For this review, take the finished solid that the model builds, in its own axes (mm). Face numbers are marked on the shaded views. Round coordinates to 2 decimals unless told otherwise and drop trailing zeros. Order: outer loops, then holes, each group sorted by start corner. A loop starts at its lowest first (then second) coordinate and runs counter-clockwise, first axis right, second up. Notation, with made-up numbers: M -31.75,18.25 L -9.75,18.25 A16 cw -9.75,34.25 Z; hole C 37,36 d3. An arc over 180 degrees is marked long. Answer in a Markdown table with one row per item. Add a question column.
Autodesk Inventor part; units mm, degrees
ref_plane "YZ Plane" through (0, 0, 0) normal (1, 0, 0) x (0, 1, 0)
ref_plane "XZ Plane" through (0, 0, 0) normal (0, 1, 0) x (-1, 0, 0)
ref_plane "XY Plane" through (0, 0, 0) normal (0, 0, 1) x (1, 0, 0)
sketch "Sketch1" plane through (0, 0, 0) normal (0, 0, 1) x (1, 0, 0)
  line L0 (0, -18) -> (0, -78)
  line L1 (0, -78) -> (19, -78)
  line L2 (19, -78) -> (19, -18)
  line L3 (19, -18) -> (0, -18)
  line L4 (19, -18) -> (447, -18)
  line L5 (447, -18) -> (447, -78)
  line L6 (447, -78) -> (19, -78)
  line L7 (447, -18) -> (466, -18)
  line L8 (466, -18) -> (466, -78)
  line L9 (466, -78) -> (447, -78)
  circle A0 centre (10, -58) radius 3
  circle A1 centre (10, -38) radius 3
  circle A2 centre (456, -58) radius 3
  circle A3 centre (456, -38) radius 3
  line L10 (19, -78) -> (19, -91)
  line L11 (19, -91) -> (447, -91)
  line L12 (447, -91) -> (447, -78)
  circle A4 centre (169, -78) radius 8
  circle A5 centre (422, -78) radius 8
  dimension "d0" = 60
  dimension "d1" = 19
  dimension "d2" = 428
  dimension "d3" = 19
  dimension "d10" = 6
  dimension "d11" = 6
  dimension "d12" = 20
  dimension "d13" = 20
  dimension "d14" = 6
  dimension "d15" = 6
  dimension "d16" = 20
  dimension "d17" = 20
  dimension "d24" = 13
  dimension "d25" = 428
  dimension "d27" = 10
  dimension "d28" = 10
  dimension "d29" = 10
  dimension "d30" = 10
  dimension "d32" = 16
  dimension "d33" = 13
  dimension "d34" = 150
  dimension "d35" = 16
  dimension "d36" = 25
extrude "Extrusion1" add sketch "Sketch1" along normal blind 2 contours L3 L2 L1 L0
extrude "Extrusion2" add sketch "Sketch1" along normal blind 2 contours L4 L5 L6 A5 A4 L2 | L6 A4 A5 L12 L11 L10
extrude "Extrusion3" add sketch "Sketch1" along normal blind 2 contours L7 L8 L9 L5
bend part "Bend Part2" radius 0.5 angle 90 line through (447, -18, 0) along (0, -1, 0) centre toward (0, 0, -1) moving side (1, 0, 0) both sides no
bend part "Bend Part3" radius 0.5 angle 90 line through (19, -78, 0) along (0, 1, 0) centre toward (0, 0, -1) moving side (-1, 0, 0) both sides no
equation "\"d1\" = d3"
equation "\"d12\" = d13"
equation "\"d16\" = d13"
equation "\"d17\" = d13"
equation "\"d25\" = d2"
equation "\"d28\" = d27"
equation "\"d29\" = d27"
properties part number "Chapa de Refrigeración" material "Aluminum 1100-H14"
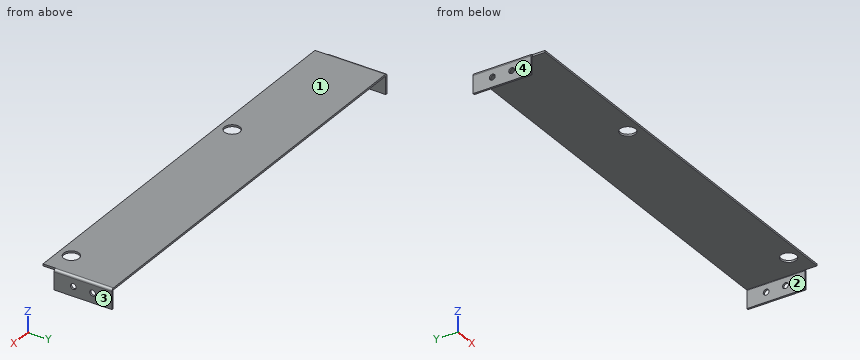
1. Consider section C-C on x = 83. Write out the cut boundary in (y, z).
2. Clearance check with flat-ended pins moving along their axes: pin 1 Ø1.6 at (y, z) = (-84.5, 1) entering from -X; pin 2 Ø3.5 at (y, z) = (-38, -8.71) entering from +X; pin 3 Ø1.2 at (x, z) = (448.5, -4.5) entering from -Y; pin 4 Ø6 at (x, y) = (350, -65) entering from -Z. State where each tip first meets the part, or that it passes through.
3. Consider section A-A on x = 422. Write out the cut boundary in (y, z), plus the area to 3 significant figures.
4. Consider section B-B on y = -74. Write out the cut boundary in (x, z), plus the area to 3 significant figures.
5. To check wall thickness, follow probe 1 along X at (y, z) = (-38, -4.25); probe 2 along Y at (x, z) = (422, 1.4); probe 3 along Z at (x, y) = (362.5, -30). State the ranges of each line that lie inside material, in increasing order. Write a range as [from, to].
6. The part is to be moulded in two halves that separate along X. For the marked faces 1, 2, 3 and 4, say which applies: pulls with the +X half, pulls with the -X half, needs draft (parallel to the pull), parting line crosses it, or undercut.
Solved:
| question | item | result |
|---|---|---|
| 1 | outline | M -91,0 L -18,0 L -18,2 L -91,2 Z |
| 2 | pin 1 | stops at x = 19 |
| 2 | pin 2 | passes through |
| 2 | pin 3 | stops at y = -78 |
| 2 | pin 4 | stops at z = 0 |
| 3 | outline | M -91,0 L -86,0 L -86,2 L -91,2 Z; M -70,0 L -18,0 L -18,2 L -70,2 Z |
| 3 | area | 114 mm^2 |
| 4 | outline | M 16.5,-18.71 L 18.5,-18.71 L 18.5,-0.5 A0.5 cw 19,0 L 162.07,0 L 162.07,2 L 19,2 A2.5 ccw 16.5,-0.5 Z; M 175.93,0 L 415.07,0 L 415.07,2 L 175.93,2 Z; M 428.93,0 L 447,0 A0.5 cw 447.5,-0.5 L 447.5,-18.71 L 449.5,-18.71 L 449.5,-0.5 A2.5 ccw 447,2 L 428.93,2 Z |
| 4 | area | 883 mm^2 |
| 5 | probe 1 | x = [16.5, 18.5], [447.5, 449.5] |
| 5 | probe 2 | y = [-91, -86], [-70, -18] |
| 5 | probe 3 | z = [0, 2] |
| 6 | face 1 | needs draft |
| 6 | face 2 | undercut |
| 6 | face 3 | pulls with the +X half |
| 6 | face 4 | pulls with the -X half |
